```python
from build123d import *

# Parameters (mm, degrees)
SKETCH_6_W          = 14
SKETCH_6_H          = 14
SKETCH_6_W_2        = 12
SKETCH_6_H_2        = 12
EXTRUDE_3_DEPTH     = 1.5
SKETCH_7_W          = 3
SKETCH_7_H          = 1.5
EXTRUDE_4_DEPTH     = 3.5
CUT_EXTRUDE_3_DEPTH = 4
SKETCH_11_R         = 1
CUT_EXTRUDE_5_DEPTH = 4
SKETCH_12_W         = 12
SKETCH_12_H         = 1
EXTRUDE_5_DEPTH     = 1


with BuildPart() as part:
    # 草图6 → 凸台-拉伸3 (new body)
    with BuildSketch(Plane.XY):
        Rectangle(SKETCH_6_W, SKETCH_6_H)
        Rectangle(SKETCH_6_W_2, SKETCH_6_H_2, mode=Mode.SUBTRACT)
    extrude(amount=EXTRUDE_3_DEPTH)

    # 草图7 → 凸台-拉伸4 (add)
    with BuildSketch(Plane.XZ.offset(7)):
        with Locations((0, 0.75)):
            Rectangle(SKETCH_7_W, SKETCH_7_H)
    extrude_4 = extrude(amount=EXTRUDE_4_DEPTH)

    # 草图8 → 切除-拉伸3 (cut)
    with BuildSketch(Plane.XY.offset(1.5)):
        with BuildLine():
            ThreePointArc((0, -10.5), (-1.060660172, -10.060660172), (-1.5, -9))
            Line((-1.5, -9), (-1.5, -10.5))
            Line((-1.5, -10.5), (0, -10.5))
        make_face()
        with BuildLine():
            Line((1.5, -10.5), (1.5, -9))
            ThreePointArc((1.5, -9), (1.060660172, -10.060660172), (0, -10.5))
            Line((0, -10.5), (1.5, -10.5))
        make_face()
    cut_extrude_3 = extrude(amount=-CUT_EXTRUDE_3_DEPTH, mode=Mode.SUBTRACT)

    # 草图11 → 切除-拉伸5 (cut)
    with BuildSketch(Plane.XY.offset(1.5)):
        with Locations((0, -9)):
            Circle(SKETCH_11_R)
    cut_extrude_5 = extrude(amount=-CUT_EXTRUDE_5_DEPTH, mode=Mode.SUBTRACT)

    # 镜向1: 凸台-拉伸4, 切除-拉伸3, 切除-拉伸5 across plane
    add(extrude_4.mirror(Plane.ZX))
    add(cut_extrude_3.mirror(Plane.ZX), mode=Mode.SUBTRACT)
    add(cut_extrude_5.mirror(Plane.ZX), mode=Mode.SUBTRACT)

    # 草图12 → 凸台-拉伸5 (add)
    with BuildSketch(Plane.XY.offset(1.5)):
        Rectangle(SKETCH_12_W, SKETCH_12_H)
    extrude(amount=-EXTRUDE_5_DEPTH)


solid = part.part
```
Work out the finished part from the listing and answer in its coordinate system (mm). A direction names the side the tool comes from. Give positions to 0.01 mm unless a question says otherwise; leave off trailing zeros. Loops run counter-clockwise (first coordinate to the right, second up) from the corner with the lowest first, then second, coordinate; pieces in that order, holes last. Notation, with made-up numbers: (28, 10) - (80, 10) arc R31 cw to (80, 39) - close; hole circle Ø9 at (10.25, 66.25). An arc over 180 degrees is marked (long way). One line per question, with ' | ' between items.
(1) Each of these flat-tipped pins is pushed along its axis until it touches: pin 1 Ø0.8 at (x, z) = (-0.5, 1) entering from -Y; pin 2 Ø0.8 at (y, z) = (7.5, 1) entering from +X; pin 3 Ø1.5 at (x, y) = (5.5, 3) entering from +Z; pin 4 Ø5 at (x, y) = (-2.5, 0.5) entering from -Z. Where does it stop, or does it pass through?
Recorded:
pin 1: stops at y = -10.5 | pin 2: stops at x = 1.5 | pin 3: stops at z = 1.5 | pin 4: stops at z = 0.5
(2) Straight lines are drawn through the part: probe 1 along Y at (x, z) = (-4, 1.25); probe 2 along Y at (x, z) = (0, 0.65); probe 3 along Y at (x, z) = (2, 0.15). For each, find the intervals that lie inside material, in ascending order.
Recorded:
probe 1: y = -7 to -6, -0.5 to 0.5, 6 to 7 | probe 2: y = -10.5 to -10, -8 to -6, -0.5 to 0.5, 6 to 8, 10 to 10.5 | probe 3: y = -7 to -6, 6 to 7
(3) The part is cut by section C-C (z = 1). Write down the section's boundary in (x, y).
Recorded:
outline: (-7, -7) - (-1.5, -7) - (-1.5, -9) arc R1.5 ccw to (1.5, -9) - (1.5, -7) - (7, -7) - (7, 7) - (1.5, 7) - (1.5, 9) arc R1.5 ccw to (-1.5, 9) - (-1.5, 7) - (-7, 7) - close; hole (-6, -6) - (6, -6) - (6, -0.5) - (-6, -0.5) - close; hole (-6, 0.5) - (6, 0.5) - (6, 6) - (-6, 6) - close; hole circle Ø2 at (0, -9); hole circle Ø2 at (0, 9)
(4) The mould has two halves that part along X. Classify faces 6 (the face through (1.5, 8, 1)), 7 (the face through (-7, 0, 1)), 8 (the face through (0, 8, 1)): +X half, -X half, draft (parallel to the pull), parting line (faces both ways), or undercut.
Recorded:
face 6: +X half | face 7: -X half | face 8: undercut
(5) The part is cut by section B-B (y = 4). Write down the section's boundary in (x, z), then the cut area to 3 significant figures.
Recorded:
outline: (-7, 0) - (-6, 0) - (-6, 1.5) - (-7, 1.5) - close; (6, 0) - (7, 0) - (7, 1.5) - (6, 1.5) - close | area: 3.00 mm²
(6) The part is cut by section A-A (x = -4.75). Write down the section's boundary in (y, z), then the cut area to 3 significant figures.
Recorded:
outline: (-7, 0) - (-6, 0) - (-6, 1.5) - (-7, 1.5) - close; (-0.5, 0.5) - (0.5, 0.5) - (0.5, 1.5) - (-0.5, 1.5) - close; (6, 0) - (7, 0) - (7, 1.5) - (6, 1.5) - close | area: 4.00 mm²
(7) A tool of negligible diameter and unlimited length cuts with its end or side. For faces 1 (the face through (0, -6, 1)), 2 (the face through (-1.5, 8, 1)), 3 (the face through (1.5, -8, 1)), 4 (the face through (4, 7, 1)), 5 (the face through (-1.5, -8, 1)), from which of +Z, -Z, +X, -X, +Y, -Y can it reach the whole face along a straight path? Write none if from no direction.
Recorded:
face 1: +Z, -Z | face 2: +Z, -Z, -X, +Y | face 3: +Z, -Z, +X, -Y | face 4: +Z, -Z, +X, +Y | face 5: +Z, -Z, -X, -Y
